Source: three-view drawing plus pictorial views. Frame: mm from the lowest corner of the part. A direction names the side the tool comes from. Coordinates: 2 decimals unless noted, no trailing zeros. Write each loop counter-clockwise with the first axis right and the second up, starting at its lowest first coordinate (ties: lowest second). Pieces come first, ordered by that corner, then holes. Notation, with made-up numbers: (3, 3.25) - (43, 3.25) arc R29 cw to (43, 35.25) - close; hole circle Ø8 at (-20, 83.25). An arc over 180 degrees is marked (long way). Put each result on its own line as item: value.
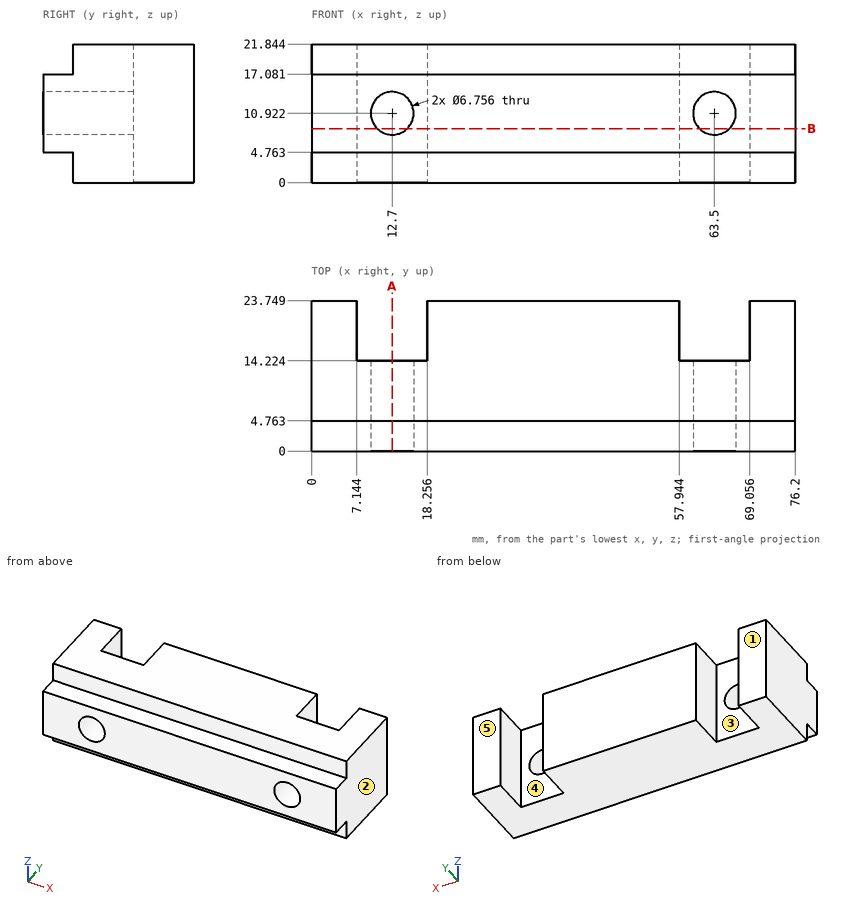
1. Section query B-B (z = 8.5). Count the separate pieces of the cut face and the enclosed holes in it, then the cut area to 3 significant figures.
Answer below:
separate pieces: 3
enclosed holes: 0
area: 1,460 mm²
2. Mould query, pull axis X, two halves, no side actions, for the marked faces 1, 2 and 3. Classes: +X half, -X half, draft (parallel to the pull), parting line (faces both ways), or undercut.
Answer below:
face 1: draft
face 2: +X half
face 3: undercut
3. Section query A-A (x = 12.7). Return loops of the section in (y, z) (1 decimal), then the cut area to 3 significant figures.
Answer below:
outline: (0, 4.8) - (4.8, 4.8) - (4.8, 0) - (14.2, 0) - (14.2, 7.5) - (0, 7.5) - close; (0, 14.3) - (14.2, 14.3) - (14.2, 21.8) - (4.8, 21.8) - (4.8, 17.1) - (0, 17.1) - close
area: 169 mm²
4. Ray query, probe 1 along X at (y, z) = (20, 15.5); probe 2 along Z at (x, y) = (12.7, 11.25) (1 decimal); probe 3 along X at (y, z) = (9.25, 9.25) (1 decimal). Return the intervals inside material, ascending. Write a range as from..to.
Answer below:
probe 1: x = 0..7.14, 18.26..57.94, 69.06..76.2
probe 2: z = 0..7.5, 14.3..21.8
probe 3: x = 0..9.8, 15.6..60.6, 66.4..76.2
5. Pin query (flat end, axial travel): pin 1 Ø3.5 at (x, z) = (64.5, 14.5) entering from +Y; pin 2 Ø1.4 at (x, y) = (39, 3) entering from -Z; pin 3 Ø1.4 at (x, z) = (27.5, 3.5) entering from -Y. Return the tip coordinate at first contact, or that it passes through.
Answer below:
pin 1: stops at y = 14.22
pin 2: stops at z = 4.76
pin 3: stops at y = 4.76
6. Set-up query: the marked faces 4 and 5. Return all of +Z, -Z, +X, -X, +Y, -Y with unobstructed straight access to the full face (end or side cutting, diameter ignored); none if empty.
Answer below:
face 4: +Z, -Z, +Y
face 5: +Z, -Z, +X, -X, +Y
